```python
from build123d import *

# Parameters (mm, degrees)
SKETCH1_R                = 8.3
SKETCH1_R_2              = 6.3
BOSS_EXTRUDE1_DEPTH      = 95
SKETCH3_R                = 8.3
BOSS_EXTRUDE2_DEPTH      = 3
SKETCH5_W                = 16.6
SKETCH5_H                = 16.6
BOSS_EXTRUDE4_DEPTH      = 7
CUT_EXTRUDE1_DEPTH       = 107.627623063
FILLET1_R                = 4.1
SKETCH4_R                = 6.3
SKETCH4_R_2              = 1.5
CUT_EXTRUDE3_DEPTH       = 3
BOSS_EXTRUDE6_START      = 2
SKETCH8_R                = 1.5
BOSS_EXTRUDE6_DEPTH      = 2
BOSS_EXTRUDE7_START      = -0.774045
BOSS_EXTRUDE7_DEPTH      = 7.774045
F_3_0_3_DIAMETER_HOLE1_D = 3
F_3_0_3_DIAMETER_HOLE2_D = 3
F_3_0_3_DIAMETER_HOLE3_D = 3


with BuildPart() as part:
    # Sketch1 → Boss-Extrude1 (new body)
    with BuildSketch(Plane(origin=(0, 0, 0), x_dir=(1, 0, 0), z_dir=(0, 1, 0))):
        with Locations(Location((0, 0, 0), (0, 0, 270))):
            Circle(SKETCH1_R)
        with Locations(Location((0, 0, 0), (0, 0, 270))):
            Circle(SKETCH1_R_2, mode=Mode.SUBTRACT)
    extrude(amount=BOSS_EXTRUDE1_DEPTH)

    # Sketch3 → Boss-Extrude2 (add)
    with BuildSketch(Plane(origin=(0, 95, 0), x_dir=(1, 0, 0), z_dir=(0, 1, 0))):
        with Locations(Location((0, 0, 0), (0, 0, 270))):
            Circle(SKETCH3_R)
    extrude(amount=BOSS_EXTRUDE2_DEPTH)

    # Sketch5 → Boss-Extrude4 (add)
    with BuildSketch(Plane(origin=(0, 98, 0), x_dir=(1, 0, 0), z_dir=(0, 1, 0))):
        Rectangle(SKETCH5_W, SKETCH5_H)
    extrude(amount=BOSS_EXTRUDE4_DEPTH)

    # Sketch6 → Cut-Extrude1 (cut, through all)
    with BuildSketch(Plane.XY.offset(8.3)):
        Polygon((4.1, 10), (0, 10), (-4.1, 10), (-4.1, 88), (4.1, 88), align=None)
    extrude(amount=-CUT_EXTRUDE1_DEPTH, mode=Mode.SUBTRACT)

    # Fillet1
    fillet1_edges = [part.edges().sort_by_distance(p)[0] for p in [
        (4.1, 88, 5.999975859),
        (4.1, 88, -5.999975859),
        (-4.1, 88, 5.999975859),
        (-4.1, 88, -5.999975859),
        (4.1, 10, -5.999975859),
        (4.1, 10, 5.999975859),
        (-4.1, 10, -5.999975859),
        (-4.1, 10, 5.999975859),
    ]]
    fillet(fillet1_edges, radius=FILLET1_R - 0.0001)  # a hair under: the kernel refuses the full size

    # Sketch4 → Cut-Extrude3 (cut)
    with BuildSketch(Plane(origin=(0, 95, 0), x_dir=(-1, 0, 0), z_dir=(0, -1, 0))):
        with Locations(Location((0, 0, 0), (0, 0, 90))):
            Circle(SKETCH4_R)
        with Locations(Location((0, 0, 0), (0, 0, 90))):
            Circle(SKETCH4_R_2, mode=Mode.SUBTRACT)
    extrude(amount=-CUT_EXTRUDE3_DEPTH, mode=Mode.SUBTRACT)

    # Sketch8 → Boss-Extrude6 (add)
    with BuildSketch(Plane(origin=(0, 95, 0), x_dir=(-1, 0, 0), z_dir=(0, -1, 0)).offset(BOSS_EXTRUDE6_START)):
        with Locations(Location((0, 0, 0), (0, 0, 90))):
            Circle(SKETCH8_R)
    extrude(amount=-BOSS_EXTRUDE6_DEPTH)

    # Sketch9 → Boss-Extrude7 (add)
    with BuildSketch(Plane.ZY.offset(8.3).offset(BOSS_EXTRUDE7_START)):
        Polygon((0, 0), (3.5, 0), (3.5, 105), (-3.5, 105), (-3.5, 0), align=None)
    boss_extrude7 = extrude(amount=BOSS_EXTRUDE7_DEPTH)

    # Mirror1: Boss-Extrude7 across plane
    add(boss_extrude7.mirror(Plane(origin=(0, 0, 0), x_dir=(0, 0, 1), z_dir=(1, 0, 0))))

    # Ø3.0 (3) Diameter Hole1 (through all)
    with Locations(Plane.XY.offset(8.3)):
        with Locations((0, 101.5)):
            Hole(F_3_0_3_DIAMETER_HOLE1_D / 2)

    # Ø3.0 (3) Diameter Hole2 (through all)
    with Locations(Plane.XY.offset(3.5)):
        with Locations((11.8, 85), (11.8, 11)):
            f_3_0_3_diameter_hole2 = Hole(F_3_0_3_DIAMETER_HOLE2_D / 2)

    # Ø3.0 (3) Diameter Hole3 (through all)
    with Locations(Plane(origin=(0, 0, -3.5), x_dir=(-1, 0, 0), z_dir=(0, 0, -1))):
        with Locations((-11.8, 65), (-11.8, 51)):
            Hole(F_3_0_3_DIAMETER_HOLE3_D / 2)

    # Mirror2: Ø3.0 (3) Diameter Hole2 across plane
    add(f_3_0_3_diameter_hole2.mirror(Plane(origin=(0, 0, 0), x_dir=(0, 0, 1), z_dir=(1, 0, 0))), mode=Mode.SUBTRACT)


solid = part.part
```
Geometry check sheet. Reference: the model listing, model coordinates, mm. A direction names the side the tool comes from. Coordinates: 2 decimals unless noted, no trailing zeros. Loops run counter-clockwise (first coordinate to the right, second up) from the corner with the lowest first, then second, coordinate; pieces in that order, holes last. Notation, with made-up numbers: (-31, -7.5) -> (-23, -7.5) arc R9 cw to (-23, 3.5) -> close; hole circle Ø11 at (-2, 26.5). An arc over 180 degrees is marked (long way). Put each result on its own line as item: value.
1) Thickness scan on line 1 (Y direction, x = 11.8, z = -0.25); line 2 (Y direction, x = 0, z = -1); line 3 (X direction, y = 96.45, z = 0). Record the ranges inside material, lowest first.
Result set:
line 1: y = 0 to 9.5, 12.5 to 49.5, 52.5 to 63.5, 66.5 to 83.5, 86.5 to 105
line 2: y = 93 to 100, 103 to 105
line 3: x = -15.3 to -6.3, -1.5 to 1.5, 6.3 to 15.3
2) Cross-section at A-A on y = 96.5. Record the boundary of the cut face in (x, z), plus the area to 3 significant figures.
Result set:
outline: (-15.3, -3.5) -> (-7.53, -3.5) arc R8.3 ccw to (7.53, -3.5) -> (15.3, -3.5) -> (15.3, 3.5) -> (7.53, 3.5) arc R8.3 ccw to (-7.53, 3.5) -> (-15.3, 3.5) -> close; circle Ø3 at (0, 0); hole circle Ø12.6 at (0, 0)
area: 200 mm^2
3) Cross-section at B-B on x = -11.8. Record the boundary of the cut face in (y, z), plus the area to 3 significant figures.
Result set:
outline: (0, -3.5) -> (9.5, -3.5) -> (9.5, 3.5) -> (0, 3.5) -> close; (12.5, -3.5) -> (83.5, -3.5) -> (83.5, 3.5) -> (12.5, 3.5) -> close; (86.5, -3.5) -> (105, -3.5) -> (105, 3.5) -> (86.5, 3.5) -> close
area: 693 mm^2
4) Cross-section at C-C on y = 29. Record the boundary of the cut face in (x, z).
Result set:
outline: (-15.3, -3.5) -> (-7.53, -3.5) arc R8.3 ccw to (-4.1, -7.22) -> (-4.1, -4.78) arc R6.3 cw to (-4.1, 4.78) -> (-4.1, 7.22) arc R8.3 ccw to (-7.53, 3.5) -> (-15.3, 3.5) -> close; (4.1, -7.22) arc R8.3 ccw to (7.53, -3.5) -> (15.3, -3.5) -> (15.3, 3.5) -> (7.53, 3.5) arc R8.3 ccw to (4.1, 7.22) -> (4.1, 4.78) arc R6.3 cw to (4.1, -4.78) -> close
5) Gauge pin test, flat ends, axial feed: pin 1 Ø5.5 at (y, z) = (100.5, -7) entering from -X; pin 2 Ø8.5 at (x, y) = (-10, 27) entering from -Z; pin 3 Ø5 at (x, y) = (11.8, 85) entering from +Z. Record the tip position at first contact, or that the pin passes through.
Result set:
pin 1: stops at x = -8.3
pin 2: stops at z = -5.99
pin 3: stops at z = 3.5
6) Release check for a two-part mould opening along Z. For faces 1 (the cylindrical face through (0.45, 95.46, -1.43)), 2 (the flat face through (4.1, 49, 6)), 3 (the flat face through (-2, 101, -8.3)) record: released by +Z, released by -Z, zero draft, split by the parting line, or undercut.
Result set:
face 1: undercut
face 2: zero draft
face 3: released by -Z
7) Tool access check on faces 4 (the flat face through (6, 98, 7)), 5 (the cylindrical face through (5.795, 48.314, -5.942)), 6 (the flat face through (4.1, 49, -6)), 7 (the cylindrical face through (-5.795, 48.314, 5.942)). Record the directions out of +Z, -Z, +X, -X, +Y, -Y that give a thin tool (end or side, any length) a straight path to the whole face; none if there is none.
Result set:
face 4: +Z, +X, -Y
face 5: -Z, -Y
face 6: +Z, -Z
face 7: +Z, -Y
8) Cross-section at D-D on x = 11.8. Record the boundary of the cut face in (y, z), plus the area to 3 significant figures.
Result set:
outline: (0, -3.5) -> (9.5, -3.5) -> (9.5, 3.5) -> (0, 3.5) -> close; (12.5, -3.5) -> (49.5, -3.5) -> (49.5, 3.5) -> (12.5, 3.5) -> close; (52.5, -3.5) -> (63.5, -3.5) -> (63.5, 3.5) -> (52.5, 3.5) -> close; (66.5, -3.5) -> (83.5, -3.5) -> (83.5, 3.5) -> (66.5, 3.5) -> close; (86.5, -3.5) -> (105, -3.5) -> (105, 3.5) -> (86.5, 3.5) -> close
area: 651 mm^2
